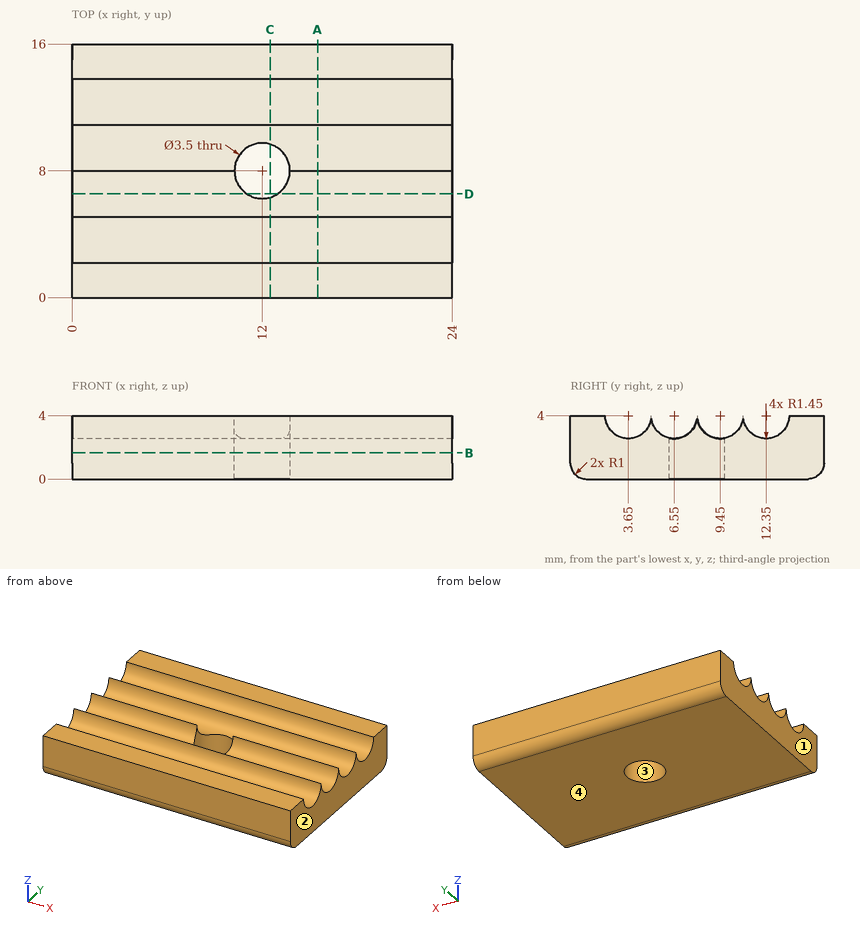
Check sheet for the drawn part. Datum: minimum x, y, z corner. Units: mm. Coordinates: 2 decimals unless noted, no trailing zeros. Write each loop counter-clockwise with the first axis right and the second up, starting at its lowest first coordinate (ties: lowest second). Pieces come first, ordered by that corner, then holes. Notation, with made-up numbers: M 13.5,55 L 54.5,55 A13 ccw 54.5,71 Z; hole C -4,-9.75 d4. An arc over 180 degrees is marked long. Use a Markdown table: item, result.
Q1. Sectioned sample at D-D, the plane y = 6.55. Record the boundary of the cut face in (x, z), plus the area to 3 significant figures.
Reply:
| item | result |
|---|---|
| outline | M 0,0 L 11.02,0 L 11.02,2.55 L 0,2.55 Z; M 12.98,0 L 24,0 L 24,2.55 L 12.98,2.55 Z |
| area | 56.2 mm² |
Q2. Sectioned sample at A-A, the plane x = 15.5. Record the boundary of the cut face in (y, z).
Reply:
| item | result |
|---|---|
| outline | M 0,1 A1 ccw 1,0 L 15,0 A1 ccw 16,1 L 16,4 L 13.8,4 A1.45 cw 10.9,4 A1.45 cw 8,4 A1.45 cw 5.1,4 A1.45 cw 2.2,4 L 0,4 Z |
Q3. Sectioned sample at B-B, the plane z = 1.65. Record the boundary of the cut face in (x, y).
Reply:
| item | result |
|---|---|
| outline | M 0,0 L 24,0 L 24,16 L 0,16 Z; hole C 12,8 d3.5 |
Q4. Thickness scan on line 1 (X direction, y = 8, z = 2.25); line 2 (Y direction, x = 3.5, z = 2.9); line 3 (Y direction, x = 6, z = 3.4). Record the ranges inside material, lowest first.
Reply:
| item | result |
|---|---|
| line 1 | x = 0 to 10.25, 13.75 to 24 |
| line 2 | y = 0 to 2.71, 4.59 to 5.61, 7.49 to 8.51, 10.39 to 11.41, 13.29 to 16 |
| line 3 | y = 0 to 2.33, 4.97 to 5.23, 7.87 to 8.13, 10.77 to 11.03, 13.67 to 16 |
Q5. Draft check along X on the marked faces 1, 2, 3 and 4. Enter one of: +X half, -X half, draft (parallel to the pull), parting line (faces both ways), or undercut.
Reply:
| item | result |
|---|---|
| face 1 | -X half |
| face 2 | +X half |
| face 3 | undercut |
| face 4 | draft |
Q6. Sectioned sample at C-C, the plane x = 12.5. Record the boundary of the cut face in (y, z).
Reply:
| item | result |
|---|---|
| outline | M 0,1 A1 ccw 1,0 L 6.32,0 L 6.32,2.57 A1.45 cw 5.1,4 A1.45 cw 2.2,4 L 0,4 Z; M 9.68,0 L 15,0 A1 ccw 16,1 L 16,4 L 13.8,4 A1.45 cw 10.9,4 A1.45 cw 9.68,2.57 Z |
